Verification items for the finished model (mm, model axes). A direction names the side the tool comes from. Give positions to 0.01 mm unless a question says otherwise; leave off trailing zeros. Order: outer loops, then holes, each group sorted by start corner. A loop starts at its lowest first (then second) coordinate and runs counter-clockwise, first axis right, second up. Notation, with made-up numbers: (44.25, 80) -> (76.25, 80) arc R4 ccw to (76.25, 87) -> close; hole circle Ø6 at (13, 68.5). An arc over 180 degrees is marked (long way). One line per question, with ' | ' between items. Start each with the question number.
Q1. Material ranges on probe 1 along X at (y, z) = (-9, 4); probe 2 along Y at (x, z) = (25.75, 4.25); probe 3 along X at (y, z) = (-10.5, 21.5), recorded low to high. Write a range as [from, to].
Q2. Go/stop test with flat-tipped pins: pin 1 (3 mm diameter, centred on y = -13.5, z = 3, fed in from +X); pin 2 (3 mm diameter, centred on x = 12.5, z = 18.5, fed in from +Y); pin 3 (3 mm diameter, centred on x = 11.5, z = 20.5, fed in from -Y); pin 4 (2 mm diameter, centred on y = -15.5, z = 9, fed in from -X). Record where each tip stops, or that it passes through.
Q3. Mould release check, pull along Y, two halves, no side actions. Record for faces 1 (the flat face through (11, -13.5, 16)), 2 (the flat face through (12, 0, 3)), 3 (the flat face through (25, -27, 3)), 4 (the flat face through (23, -32, 3)): released by +Y, released by -Y, zero draft, split by the parting line, or undercut.
Q4. Section check D-D on y = -9.5. Record the cut outline in (x, z).
Q5. Access from +Z, -Z, +X, -X, +Y, -Y to the whole of each face (thin tool, end or side, straight path). Record for faces 5 (the flat face through (9.5, -10, 16)), 6 (the flat face through (27, -13, 3)), 7 (the flat face through (27, -24, 3)), 8 (the flat face through (13.5, -27, 16)).
Q6. Section check A-A on z = 13.5. Record the cut outline in (x, y).
Q7. Section check B-B on y = -25.5. Record the cut outline in (x, z), plus the area to 3 significant figures.
Q8. Section check C-C on x = 10.25. Record the cut outline in (y, z), plus the area to 3 significant figures.
from build123d import *

# Parameters (mm, degrees)
F0_W     = 4
F0_H     = 7
F0_W_2   = 3
F0_H_2   = 5
F1_DEPTH = 6
F2_DEPTH = 26


with BuildPart() as f1:
    # F0 (on Top) → F1 (new body)
    with BuildSketch(Plane.XY):
        Polygon((23, 0), (0, 0), (0, -37), (23, -37), (23, -27), (23, -10), align=None)
        with Locations((11.5, -27)):
            Rectangle(F0_W, F0_H, mode=Mode.SUBTRACT)
        with Locations((11.5, -10)):
            Rectangle(F0_W, F0_H, mode=Mode.SUBTRACT)
        Polygon((27, -10), (23, -10), (23, -27), (27, -27), (27, -21), (27, -16), align=None)
        with Locations((28.5, -18.5)):
            Rectangle(F0_W_2, F0_H_2)
    extrude(amount=F1_DEPTH)

    # F0 (on Top) → F2 (join)
    with BuildSketch(Plane.XY):
        with Locations((11.5, -10)):
            Rectangle(F0_W, F0_H)
        with Locations((11.5, -27)):
            Rectangle(F0_W, F0_H)
    extrude(amount=F2_DEPTH)


solid = f1.part
Filled in:
1) probe 1: [0, 23] | probe 2: [-27, -10] | probe 3: [9.5, 13.5]
2) pin 1: x = 27 | pin 2: y = -6.5 | pin 3: y = -30.5 | pin 4: through
3) face 1: undercut | face 2: released by +Y | face 3: released by -Y | face 4: zero draft
4) outline: (0, 0) -> (23, 0) -> (23, 6) -> (13.5, 6) -> (13.5, 26) -> (9.5, 26) -> (9.5, 6) -> (0, 6) -> close
5) face 5: +Z, -X, +Y, -Y | face 6: +Z, -Z, +X, +Y | face 7: +Z, -Z, +X, -Y | face 8: +Z, +X, +Y, -Y
6) outline: (9.5, -30.5) -> (13.5, -30.5) -> (13.5, -23.5) -> (9.5, -23.5) -> close; (9.5, -13.5) -> (13.5, -13.5) -> (13.5, -6.5) -> (9.5, -6.5) -> close
7) outline: (0, 0) -> (27, 0) -> (27, 6) -> (13.5, 6) -> (13.5, 26) -> (9.5, 26) -> (9.5, 6) -> (0, 6) -> close | area: 242 mm²
8) outline: (-37, 0) -> (0, 0) -> (0, 6) -> (-6.5, 6) -> (-6.5, 26) -> (-13.5, 26) -> (-13.5, 6) -> (-23.5, 6) -> (-23.5, 26) -> (-30.5, 26) -> (-30.5, 6) -> (-37, 6) -> close | area: 502 mm²
